Autodesk Inventor part; units mm, degrees
ref_plane "YZ Plane" through (0, 0, 0) normal (1, 0, 0) x (0, 1, 0)
ref_plane "XZ Plane" through (0, 0, 0) normal (0, 1, 0) x (-1, 0, 0)
ref_plane "XY Plane" through (0, 0, 0) normal (0, 0, 1) x (1, 0, 0)
sketch "Sketch1" plane through (0, 0, 0) normal (0, 0, 1) x (1, 0, 0)
  line L0 (0, 0) -> (157, 0)
  line L1 (157, 0) -> (157, 10)
  line L2 (157, 10) -> (0, 10)
  line L3 (0, 10) -> (0, 0)
  circle A0 centre (47.5, 5) radius 1.6
  circle A1 centre (107.5, 5) radius 1.6
  circle A2 centre (152, 5) radius 1.6
  circle A3 centre (142.5, 5) radius 1.6
  circle A4 centre (5, 5) radius 1.6
  circle A5 centre (14, 5) radius 1.6
  dimension "d1" = 10
  dimension "d2" = 90
  dimension "d4" = 3.2
  dimension "d6" = 3.2
  dimension "d7" = 3.2
  dimension "d8" = 60
  dimension "d9" = 44.5
  dimension "d26" = 3.2
  dimension "d27" = 35
  dimension "d28" = 3.2
  dimension "d29" = 42.5
  dimension "d32" = 5
  dimension "d33" = 5
  dimension "d34" = 3.2
  dimension "d35" = 9
ref_plane "Work Plane2" through (0, 0, 0) normal (0, -1, 0) x (1, 0, 0)
sketch "Sketch2" plane through (0, 0, 0) normal (0, -1, 0) x (1, 0, 0)
  circle A0 centre (42.5, 7) radius 1.6
  circle A1 centre (112.5, 7) radius 1.6
  circle A2 centre (77.5, 7) radius 1.6
  dimension "d13" = 3.2
  dimension "d15" = 3.2
  dimension "d16" = 70
  dimension "d17" = 3.2
  dimension "d18" = 35
ref_plane "Work Plane1" through (0, 0, 11) normal (0, 0, 1) x (1, 0, 0)
extrude "Extrusion4" add sketch "Sketch1" along normal blind 11
extrude "Extrusion5" cut sketch "Sketch2" against normal up to next
sketch "Sketch7" plane through (0, 0, 0) normal (0, -1, 0) x (1, 0, 0)
  line L0 (0, 11) -> (0, 5)
  line L1 (0, 11) -> (25, 11)
  line L2 (25, 11) -> (0, 5)
  point P0 (0, 0)
extrude "Extrusion6" cut sketch "Sketch7" against normal up to next
sketch "Sketch8" plane through (0, 0, 0) normal (0, -1, 0) x (1, 0, 0)
  line L0 (157, 11) -> (25, 11)
  line L1 (157, 11) -> (157, 5)
  line L2 (157, 0) -> (157, 11)
  line L3 (157, 0) -> (157, 11)
  line L4 (157, 11) -> (132, 11)
  line L5 (25, 11) -> (157, 11)
  line L6 (132, 11) -> (157, 5)
  point P0 (0, 0)
extrude "Extrusion7" cut sketch "Sketch8" against normal up to next
sketch "Sketch5" plane through (0, 0, 11) normal (0, 0, 1) x (1, 0, 0)
  circle A0 centre (47.5, 5) radius 1.6
  line L0 (50.9064, 5) -> (49.2032, 2.05)
  line L1 (49.2032, 2.05) -> (45.7968, 2.05)
  line L2 (45.7968, 2.05) -> (44.0936, 5)
  line L3 (44.0936, 5) -> (45.7968, 7.95)
  line L4 (45.7968, 7.95) -> (49.2032, 7.95)
  line L5 (49.2032, 7.95) -> (50.9064, 5)
  circle A1 centre (107.5, 5) radius 1.6
  line L6 (110.9064, 5) -> (109.2032, 2.05)
  line L7 (109.2032, 2.05) -> (105.7968, 2.05)
  line L8 (105.7968, 2.05) -> (104.0936, 5)
  line L9 (104.0936, 5) -> (105.7968, 7.95)
  line L10 (105.7968, 7.95) -> (109.2032, 7.95)
  line L11 (109.2032, 7.95) -> (110.9064, 5)
  dimension "d44" = 5.9
  dimension "d45" = 5.9
sketch "Sketch9" plane through (0, 0, 11) normal (0, 0, 1) x (1, 0, 0)
  circle A0 centre (14, 5) radius 1.6
  line L0 (17.4064, 5) -> (15.7032, 2.05)
  line L1 (15.7032, 2.05) -> (12.2968, 2.05)
  line L2 (12.2968, 2.05) -> (10.5936, 5)
  line L3 (10.5936, 5) -> (12.2968, 7.95)
  line L4 (12.2968, 7.95) -> (15.7032, 7.95)
  line L5 (15.7032, 7.95) -> (17.4064, 5)
  circle A1 centre (142.5, 5) radius 1.6
  line L6 (145.9064, 5) -> (144.2032, 2.05)
  line L7 (144.2032, 2.05) -> (140.7968, 2.05)
  line L8 (140.7968, 2.05) -> (139.0936, 5)
  line L9 (139.0936, 5) -> (140.7968, 7.95)
  line L10 (140.7968, 7.95) -> (144.2032, 7.95)
  line L11 (144.2032, 7.95) -> (145.9064, 5)
  point P0 (0, 0)
  dimension "d51" = 5.9
  dimension "d52" = 5.9
sketch "Sketch10" plane through (0, 0, 11) normal (0, 0, 1) x (1, 0, 0)
  line L0 (8.4064, 5) -> (6.7032, 2.05)
  line L1 (6.7032, 2.05) -> (3.2968, 2.05)
  line L2 (3.2968, 2.05) -> (1.5936, 5)
  line L3 (1.5936, 5) -> (3.2968, 7.95)
  line L4 (3.2968, 7.95) -> (6.7032, 7.95)
  line L5 (6.7032, 7.95) -> (8.4064, 5)
  line L6 (155.4064, 5) -> (153.7032, 2.05)
  line L7 (153.7032, 2.05) -> (150.2968, 2.05)
  line L8 (150.2968, 2.05) -> (148.5936, 5)
  line L9 (148.5936, 5) -> (150.2968, 7.95)
  line L10 (150.2968, 7.95) -> (153.7032, 7.95)
  line L11 (153.7032, 7.95) -> (155.4064, 5)
  point P0 (0, 0)
  point P1 (5, 5)
  point P2 (152, 5)
  dimension "d53" = 5.9
  dimension "d54" = 5.9
extrude "Extrusion8" cut sketch "Sketch5" against normal blind 3
extrude "Extrusion9" cut sketch "Sketch9" against normal blind 5
extrude "Extrusion10" cut sketch "Sketch10" against normal blind 7
properties part number "new_wheel_support_v2"
Verification items for the finished model (mm, model axes). A direction names the side the tool comes from. Coordinates: 2 decimals unless noted, no trailing zeros. Write each loop counter-clockwise with the first axis right and the second up, starting at its lowest first coordinate (ties: lowest second). Pieces come first, ordered by that corner, then holes. Notation, with made-up numbers: M 74,69 L 117,69 A20 ccw 117,91 Z; hole C 61.5,88.5 d3. An arc over 180 degrees is marked long. Answer as a JSON object with one key per item and string values. Group by question number.
(1) Cross-section at A-A, the plane x = 77.5. Record the cut outline in (y, z).
(2) Release check for a two-part mould opening along Y. For faces 1 (the face through (5.86, 3.65, 1.97)), 2 (the face through (77, 0, 4)), 3 (the face through (77, 5, 0)) record: +Y half, -Y half, draft (parallel to the pull), parting line (faces both ways), or undercut.
(3) Gauge pin test, flat ends, axial feed: pin 1 (3 mm diameter, centred on x = 42.5, z = 7, fed in from +Y); pin 2 (1 mm diameter, centred on x = 107.5, y = 6.5, fed in from +Z); pin 3 (5 mm diameter, centred on x = 14, y = 5, fed in from +Z). Record the tip position at first contact, or that the pin passes through.
(4) Tool access check on faces 4 (the face through (16.57, 3.55, 7.61)), 5 (the face through (0, 5, 2)). Record the directions out of +Z, -Z, +X, -X, +Y, -Y that give a thin tool (end or side, any length) a straight path to the whole face; none if there is none.
(5) Material ranges on line 1 (Z direction, x = 42.5, y = 5.25); line 2 (Y direction, x = 142.5, z = 1.8); line 3 (Z direction, x = 43, y = 3), recorded low to high.
(6) Cross-section at D-D, the plane x = 5. Record the cut outline in (y, z), and give its area (3 significant figures).
(7) Cross-section at C-C, the plane x = 107.5. Record the cut outline in (y, z).
(8) Cross-section at B-B, the plane z = 1.5. Record the cut outline in (x, y), and give its area (3 significant figures).
Reply:
{
 "1": {"outline": "M 0,0 L 10,0 L 10,5.4 L 0,5.4 Z; M 0,8.6 L 10,8.6 L 10,11 L 0,11 Z"},
 "2": {"face 1": "undercut", "face 2": "-Y half", "face 3": "draft"},
 "3": {"pin 1": "through", "pin 2": "z = 8", "pin 3": "z = 6"},
 "4": {"face 4": "+Z", "face 5": "+Z, -Z, -X, +Y, -Y"},
 "5": {"line 1": "0 to 5.4, 8.6 to 11", "line 2": "0 to 3.4, 6.6 to 10", "line 3": "0 to 5.48, 8.52 to 11"},
 "6": {"outline": "M 0,0 L 3.4,0 L 3.4,4 L 2.05,4 L 2.05,6.2 L 0,6.2 Z; M 6.6,0 L 10,0 L 10,6.2 L 7.95,6.2 L 7.95,4 L 6.6,4 Z", "area": "36.2 mm²"},
 "7": {"outline": "M 0,0 L 3.4,0 L 3.4,8 L 2.05,8 L 2.05,11 L 0,11 Z; M 6.6,0 L 10,0 L 10,11 L 7.95,11 L 7.95,8 L 6.6,8 Z"},
 "8": {"outline": "M 0,0 L 157,0 L 157,10 L 0,10 Z; hole C 5,5 d3.2; hole C 14,5 d3.2; hole C 47.5,5 d3.2; hole C 107.5,5 d3.2; hole C 142.5,5 d3.2; hole C 152,5 d3.2", "area": "1,520 mm²"}
}
